Geometry check sheet. Reference: the model listing, model coordinates, mm. A direction names the side the tool comes from. Give positions to 0.01 mm unless a question says otherwise; leave off trailing zeros. Write each loop counter-clockwise with the first axis right and the second up, starting at its lowest first coordinate (ties: lowest second). Pieces come first, ordered by that corner, then holes. Notation, with made-up numbers: (51, -20) -> (78, -20) arc R9 ccw to (78, -11) -> close; hole circle Ø7 at (-14.5, -11). An arc over 180 degrees is marked (long way). One line per item, written item: value.
from build123d import *

# Parameters (mm, degrees)
ESQUISSE2_W                    = 50.8
ESQUISSE2_H                    = 50.8
ESQUISSE2_W_2                  = 44.45
ESQUISSE2_H_2                  = 44.45
BOSS_EXTRU_1_DEPTH             = 649.999999972
ESQUISSE4_R                    = 3.175
ENL_V_MAT_EXTRU_2_DEPTH        = 653.476666222
M4_CLEARANCE_HOLE1_D           = 4.5
M4_CLEARANCE_HOLE1_DEPTH       = 3.175
M4_CLEARANCE_HOLE1_CSINK_D     = 4.85
M4_CLEARANCE_HOLE1_CSINK_ANGLE = 90


with BuildPart() as part:
    # Esquisse2 → Boss.-Extru.1 (new, symmetric)
    with BuildSketch(Plane.XY):
        Rectangle(ESQUISSE2_W, ESQUISSE2_H)
        Rectangle(ESQUISSE2_W_2, ESQUISSE2_H_2, mode=Mode.SUBTRACT)
    extrude(amount=BOSS_EXTRU_1_DEPTH, both=True)

    # Esquisse4 → Enlèv. mat.-Extru.2 (cut, through all)
    with BuildSketch(Plane.ZY.offset(25.4)):
        with Locations((-634.999999972, 0)):
            Circle(ESQUISSE4_R)
    extrude(amount=-ENL_V_MAT_EXTRU_2_DEPTH, mode=Mode.SUBTRACT)

    # M4 Clearance Hole1
    with Locations(Plane.ZY.offset(25.4)):
        with Locations((517.099999972, -3.175), (557.099999972, -3.175), (597.099999972, -3.175)):
            CounterSinkHole(M4_CLEARANCE_HOLE1_D / 2, M4_CLEARANCE_HOLE1_CSINK_D / 2, depth=M4_CLEARANCE_HOLE1_DEPTH, counter_sink_angle=M4_CLEARANCE_HOLE1_CSINK_ANGLE)


solid = part.part
1) Scan lines: probe 1 along X at (y, z) = (-10, 476) (3 decimals); probe 2 along Y at (x, z) = (-24.5, -635) (3 decimals). Record each from-to range of solid material in increasing order.
Verdict:
probe 1: -25.4 to -22.225, 22.225 to 25.4
probe 2: -25.4 to -3.175, 3.175 to 25.4
2) Depth check by flat-ended pin: pin 1 Ø4 at (y, z) = (-3.175, 597.1) entering from -X (3 decimals); pin 2 Ø10 at (x, y) = (5, 17.5) entering from -Z. Enter the tip coordinate at first touch or a pass-through.
Verdict:
pin 1: x = 22.225
pin 2: z = -650
3) Sectioned sample at B-B on z = 468. Record the cut outline in (x, y) (3 decimals), plus the area to 3 significant figures.
Verdict:
outline: (-25.4, -25.4) -> (25.4, -25.4) -> (25.4, 25.4) -> (-25.4, 25.4) -> close; hole (-22.225, -22.225) -> (22.225, -22.225) -> (22.225, 22.225) -> (-22.225, 22.225) -> close
area: 605 mm^2
4) Sectioned sample at A-A on x = -4. Record the cut outline in (y, z) (3 decimals), plus the area to 4 significant figures.
Verdict:
outline: (-25.4, -650) -> (-22.225, -650) -> (-22.225, 650) -> (-25.4, 650) -> close; (22.225, -650) -> (25.4, -650) -> (25.4, 650) -> (22.225, 650) -> close
area: 8,255 mm^2
5) Mould release check, pull along Y, two halves, no side actions. Record for faces 3 (the flat face through (0, 25.4, 9)), 4 (the flat face through (-23, 0, -650)), 5 (the flat face through (0, 22.225, 9)): released by +Y, released by -Y, zero draft, split by the parting line, or undercut.
Verdict:
face 3: released by +Y
face 4: zero draft
face 5: undercut
6) Tool access check on faces 1 (the flat face through (-23, 0, 650)), 2 (the flat face through (0, -22.225, 9)). Record the directions out of +Z, -Z, +X, -X, +Y, -Y that give a thin tool (end or side, any length) a straight path to the whole face; none if there is none.
Verdict:
face 1: +Z, +X, -X, +Y, -Y
face 2: +Z, -Z
